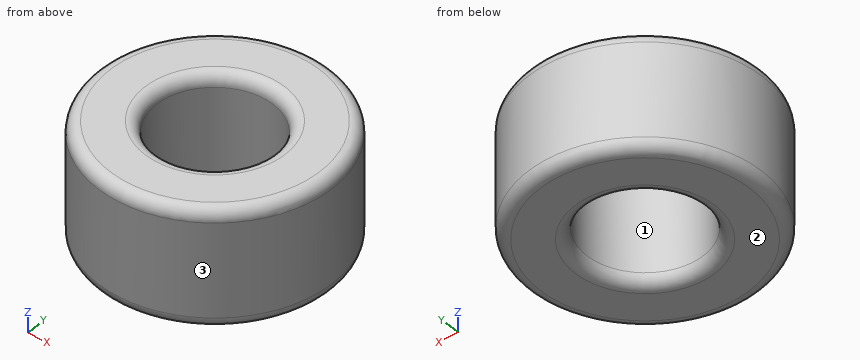
```python
from build123d import *

# Parameters (mm, degrees)
F0_R     = 50.8
F1_DEPTH = 50.8
F2_R     = 25.4
F3_DEPTH = 50.8
F4_R     = 5.08
F5_R     = 5.08


with BuildPart() as f1:
    # F0 (on Top) → F1 (new body)
    with BuildSketch(Plane.XY):
        Circle(F0_R)
    extrude(amount=-F1_DEPTH)

    # F2 (on Top) → F3 (cut)
    with BuildSketch(Plane.XY):
        Circle(F2_R)
    extrude(amount=-F3_DEPTH, mode=Mode.SUBTRACT)

    # F4
    f4_edges = [f1.edges().sort_by_distance(p)[0] for p in [
        (-50.8, 0, 0),
        (-25.4, 0, 0),
    ]]
    fillet(f4_edges, radius=F4_R)

    # F5
    f5_edges = [f1.edges().sort_by_distance(p)[0] for p in [
        (-50.8, 0, -50.8),
        (-25.4, 0, -50.8),
    ]]
    fillet(f5_edges, radius=F5_R)


solid = f1.part
```
Read the model definition and answer for the solid it produces. Units are mm, in the model's axes. Face numbers are marked on the shaded views. Coordinates: 2 decimals unless noted, no trailing zeros. Loops run counter-clockwise (first coordinate to the right, second up) from the corner with the lowest first, then second, coordinate; pieces in that order, holes last. Notation, with made-up numbers: (-31, -36) - (15, -36) arc R4 cw to (15, -29) - close; hole circle Ø4 at (23, 0.5). An arc over 180 degrees is marked (long way). Answer in a Markdown table with one row per item.
1. Find section A-A, the plane x = 0. Write down the section's boundary in (y, z).
Conclusion:
| item | result |
|---|---|
| outline | (-50.8, -45.72) arc R5.08 ccw to (-45.72, -50.8) - (-30.48, -50.8) arc R5.08 ccw to (-25.4, -45.72) - (-25.4, -5.08) arc R5.08 ccw to (-30.48, 0) - (-45.72, 0) arc R5.08 ccw to (-50.8, -5.08) - close; (25.4, -45.72) arc R5.08 ccw to (30.48, -50.8) - (45.72, -50.8) arc R5.08 ccw to (50.8, -45.72) - (50.8, -5.08) arc R5.08 ccw to (45.72, 0) - (30.48, 0) arc R5.08 ccw to (25.4, -5.08) - close |
2. Given pin 1 (8 mm diameter, centred on x = 8, z = -12.5, fed in from -Y); pin 2 (12 mm diameter, centred on x = 6.5, y = -22.5, fed in from +Z); pin 3 (5 mm diameter, centred on x = 19.5, z = -7, fed in from -Y), each flat-ended and moving along its own axis, determine where each tip first touches the part or whether it passes through.
Conclusion:
| item | result |
|---|---|
| pin 1 | stops at y = -50.64 |
| pin 2 | stops at z = -0.11 |
| pin 3 | stops at y = -47.87 |
3. Straight lines are drawn through the part: line 1 (Y direction, x = 0, z = -33); line 2 (Y direction, x = -44, z = -9); line 3 (X direction, y = -9.5, z = -21). For each, find the intervals that lie inside material, in ascending order.
Conclusion:
| item | result |
|---|---|
| line 1 | y = -50.8 to -25.4, 25.4 to 50.8 |
| line 2 | y = -25.39 to 25.39 |
| line 3 | x = -49.9 to -23.56, 23.56 to 49.9 |
4. Determine the mould class of the marked faces 1, 2 and 3 for opening direction X: +X half, -X half, draft (parallel to the pull), parting line (faces both ways), or undercut.
Conclusion:
| item | result |
|---|---|
| face 1 | undercut |
| face 2 | draft |
| face 3 | parting line |
5. Find section C-C, the plane z = -26. Write down the section's boundary in (x, y).
Conclusion:
| item | result |
|---|---|
| outline | circle Ø101.6 at (0, 0); hole circle Ø50.8 at (0, 0) |
